Check sheet for the modelled part. Datum: model origin and axes. Units: mm. A direction names the side the tool comes from. Coordinates: 2 decimals unless noted, no trailing zeros. Write each loop counter-clockwise with the first axis right and the second up, starting at its lowest first coordinate (ties: lowest second). Pieces come first, ordered by that corner, then holes. Notation, with made-up numbers: (-2, -25) -> (11, -25) arc R19 cw to (11, 10) -> close; hole circle Ø3 at (80, 10.5). An arc over 180 degrees is marked (long way). Put each result on its own line as item: value.
```python
from build123d import *

# Parameters (mm, degrees)
SKETCH_1_R        = 19
SKETCH_1_R_2      = 17
EXTRUDE_2_DEPTH   = 11
EXTRUDE_2_2_DEPTH = 11
EXTRUDE_2_3_DEPTH = 11
EXTRUDE_2_4_DEPTH = 11
EXTRUDE_2_5_DEPTH = 11
EXTRUDE_2_6_DEPTH = 11
EXTRUDE_2_7_DEPTH = 11
EXTRUDE_2_8_DEPTH = 11
SKETCH_1_8_R      = 86
SKETCH_1_8_R_2    = 19
SKETCH_1_8_R_3    = 1.55
EXTRUDE_3_DEPTH   = 3


with BuildPart() as part:
    # Sketch 1 → Extrude 2 (new body)
    with BuildSketch(Plane(origin=(0, 0, 0), x_dir=(1, 0, 0), z_dir=(0, 1, 0))):
        with Locations(Location((-63, 0, 0), (0, 0, 270))):
            Circle(SKETCH_1_R)
        with Locations(Location((-63, 0, 0), (0, 0, 270))):
            Circle(SKETCH_1_R_2, mode=Mode.SUBTRACT)
    extrude(amount=EXTRUDE_2_DEPTH)



with BuildPart() as body_2:
    # Sketch 1 → Extrude 2 2 (new body)
    with BuildSketch(Plane(origin=(0, 0, 0), x_dir=(1, 0, 0), z_dir=(0, 1, 0))):
        with Locations(Location((-44.547727215, -44.547727215, 0), (0, 0, 270))):
            Circle(SKETCH_1_R)
        with Locations(Location((-44.547727215, -44.547727215, 0), (0, 0, 270))):
            Circle(SKETCH_1_R_2, mode=Mode.SUBTRACT)
    extrude(amount=EXTRUDE_2_2_DEPTH)


with BuildPart() as body_3:
    # Sketch 1 → Extrude 2 3 (new body)
    with BuildSketch(Plane(origin=(0, 0, 0), x_dir=(1, 0, 0), z_dir=(0, 1, 0))):
        with Locations(Location((0, -63, 0), (0, 0, 270))):
            Circle(SKETCH_1_R)
        with Locations(Location((0, -63, 0), (0, 0, 270))):
            Circle(SKETCH_1_R_2, mode=Mode.SUBTRACT)
    extrude(amount=EXTRUDE_2_3_DEPTH)


with BuildPart() as body_4:
    # Sketch 1 → Extrude 2 4 (new body)
    with BuildSketch(Plane(origin=(0, 0, 0), x_dir=(1, 0, 0), z_dir=(0, 1, 0))):
        with Locations(Location((44.547727215, -44.547727215, 0), (0, 0, 270))):
            Circle(SKETCH_1_R)
        with Locations(Location((44.547727215, -44.547727215, 0), (0, 0, 270))):
            Circle(SKETCH_1_R_2, mode=Mode.SUBTRACT)
    extrude(amount=EXTRUDE_2_4_DEPTH)


with BuildPart() as body_5:
    # Sketch 1 → Extrude 2 5 (new body)
    with BuildSketch(Plane(origin=(0, 0, 0), x_dir=(1, 0, 0), z_dir=(0, 1, 0))):
        with Locations(Location((63, 0, 0), (0, 0, 270))):
            Circle(SKETCH_1_R)
        with Locations(Location((63, 0, 0), (0, 0, 270))):
            Circle(SKETCH_1_R_2, mode=Mode.SUBTRACT)
    extrude(amount=EXTRUDE_2_5_DEPTH)


with BuildPart() as body_6:
    # Sketch 1 → Extrude 2 6 (new body)
    with BuildSketch(Plane(origin=(0, 0, 0), x_dir=(1, 0, 0), z_dir=(0, 1, 0))):
        with Locations(Location((0, 63, 0), (0, 0, 270))):
            Circle(SKETCH_1_R)
        with Locations(Location((0, 63, 0), (0, 0, 270))):
            Circle(SKETCH_1_R_2, mode=Mode.SUBTRACT)
    extrude(amount=EXTRUDE_2_6_DEPTH)


with BuildPart() as body_7:
    # Sketch 1 → Extrude 2 7 (new body)
    with BuildSketch(Plane(origin=(0, 0, 0), x_dir=(1, 0, 0), z_dir=(0, 1, 0))):
        with Locations(Location((44.547727215, 44.547727215, 0), (0, 0, 270))):
            Circle(SKETCH_1_R)
        with Locations(Location((44.547727215, 44.547727215, 0), (0, 0, 270))):
            Circle(SKETCH_1_R_2, mode=Mode.SUBTRACT)
    extrude(amount=EXTRUDE_2_7_DEPTH)


with BuildPart() as body_8:
    # Sketch 1 → Extrude 2 8 (new body)
    with BuildSketch(Plane(origin=(0, 0, 0), x_dir=(1, 0, 0), z_dir=(0, 1, 0))):
        with Locations(Location((-44.544339366, 44.544339366, 0), (0, 0, 270))):
            Circle(SKETCH_1_R)
        with Locations(Location((-44.544339366, 44.544339366, 0), (0, 0, 270))):
            Circle(SKETCH_1_R_2, mode=Mode.SUBTRACT)
    extrude(amount=EXTRUDE_2_8_DEPTH)


with BuildPart() as part_1:
    add(part.part)

    add(body_2.part)  # Extrude 3 merges body 2

    add(body_3.part)  # Extrude 3 merges body 3

    add(body_4.part)  # Extrude 3 merges body 4

    add(body_5.part)  # Extrude 3 merges body 5

    add(body_6.part)  # Extrude 3 merges body 6

    add(body_7.part)  # Extrude 3 merges body 7

    add(body_8.part)  # Extrude 3 merges body 8
    # Sketch 1_8 → Extrude 3 (add)
    with BuildSketch(Plane(origin=(0, 0, 0), x_dir=(1, 0, 0), z_dir=(0, 1, 0))):
        with Locations(Location((0, 0, 0), (0, 0, 270))):
            Circle(SKETCH_1_8_R)
        with Locations(Location((-63, 0, 0), (0, 0, 270))):
            Circle(SKETCH_1_8_R_2, mode=Mode.SUBTRACT)
        with Locations(Location((-44.547727215, -44.547727215, 0), (0, 0, 270))):
            Circle(SKETCH_1_8_R_2, mode=Mode.SUBTRACT)
        with Locations(Location((0, -63, 0), (0, 0, 270))):
            Circle(SKETCH_1_8_R_2, mode=Mode.SUBTRACT)
        with Locations(Location((44.547727215, -44.547727215, 0), (0, 0, 270))):
            Circle(SKETCH_1_8_R_2, mode=Mode.SUBTRACT)
        with Locations(Location((63, 0, 0), (0, 0, 270))):
            Circle(SKETCH_1_8_R_2, mode=Mode.SUBTRACT)
        with Locations(Location((44.547727215, 44.547727215, 0), (0, 0, 270))):
            Circle(SKETCH_1_8_R_2, mode=Mode.SUBTRACT)
        with Locations(Location((0, 63, 0), (0, 0, 270))):
            Circle(SKETCH_1_8_R_2, mode=Mode.SUBTRACT)
        with Locations(Location((-44.544339366, 44.544339366, 0), (0, 0, 270))):
            Circle(SKETCH_1_8_R_2, mode=Mode.SUBTRACT)
        with Locations(Location((0, -7, 0), (0, 0, 270))):
            Circle(SKETCH_1_8_R_3, mode=Mode.SUBTRACT)
        with Locations(Location((-7, 0, 0), (0, 0, 270))):
            Circle(SKETCH_1_8_R_3, mode=Mode.SUBTRACT)
        with Locations(Location((7, 0, 0), (0, 0, 270))):
            Circle(SKETCH_1_8_R_3, mode=Mode.SUBTRACT)
        with Locations(Location((0, 7, 0), (0, 0, 270))):
            Circle(SKETCH_1_8_R_3, mode=Mode.SUBTRACT)
        with Locations(Location((0, 0, 0), (0, 0, 270))):
            Circle(SKETCH_1_8_R_3, mode=Mode.SUBTRACT)
    extrude(amount=EXTRUDE_3_DEPTH)


solid = part_1.part
```
Q1. Cross-section at C-C (x = 30). Record the cut outline in (y, z), plus the area to 3 significant figures.
Recorded:
outline: (0, -80.6) -> (3, -80.6) -> (3, -56.77) -> (11, -56.77) -> (11, -53.34) -> (0, -53.34) -> close; (0, -35.75) -> (11, -35.75) -> (11, -32.33) -> (3, -32.33) -> (3, 32.33) -> (11, 32.33) -> (11, 35.75) -> (0, 35.75) -> close; (0, 53.34) -> (11, 53.34) -> (11, 56.77) -> (3, 56.77) -> (3, 80.6) -> (0, 80.6) -> close
area: 488 mm2
Q2. Material ranges on line 1 along X through (y, z) = (1.75, 35); line 2 along X through (y, z) = (9, 7.5); line 3 along X through (y, z) = (5.5, -29), recorded low to high.
Recorded:
line 1: x = -78.56 to -58.61, -30.48 to 30.48, 58.61 to 78.56
line 2: x = -80.46 to -78.26, -47.74 to -45.54, 45.54 to 47.74, 78.26 to 80.46
line 3: x = -55.47 to -51.43, -37.66 to -33.62, 33.63 to 37.67, 51.42 to 55.47
Q3. Cross-section at D-D (x = -57). Record the cut outline in (y, z), plus the area to 3 significant figures.
Recorded:
outline: (0, -64.4) -> (3, -64.4) -> (3, -58.89) -> (11, -58.89) -> (11, -56.11) -> (0, -56.11) -> close; (0, -32.97) -> (11, -32.97) -> (11, -30.2) -> (3, -30.2) -> (3, -18.03) -> (11, -18.03) -> (11, -15.91) -> (0, -15.91) -> close; (0, 15.91) -> (11, 15.91) -> (11, 18.03) -> (3, 18.03) -> (3, 30.2) -> (11, 30.2) -> (11, 32.97) -> (0, 32.97) -> close; (0, 56.12) -> (11, 56.12) -> (11, 58.9) -> (3, 58.9) -> (3, 64.4) -> (0, 64.4) -> close
area: 275 mm2
Q4. Depth check by flat-ended pin: P1, Ø3.5, axis at x = 0, z = 7, coming from the +Y side; P2, Ø3.5, axis at x = -7, z = 0, coming from the -Y side; P3, Ø6, axis at y = 1.5, z = -45, coming from the +X side; P4, Ø1.5, axis at y = 9, z = 35.5, coming from the +X side. Enter the tip coordinate at first touch or a pass-through.
Recorded:
P1: stops at y = 3
P2: stops at y = 0
P3: stops at x = 75.05
P4: stops at x = 61.64
Q5. Mould release check, pull along X, two halves, no side actions. Record for faces 3 (the cylindrical face through (57.389, 6.944, 30.544)), 4 (the cylindrical face through (57.39, 6.94, -58.55)), 5 (the flat face through (35, 11, 30)): released by +X, released by -X, zero draft, split by the parting line, or undercut.
Recorded:
face 3: undercut
face 4: undercut
face 5: zero draft
Q6. Cross-section at B-B (z = -70.5). Record the cut outline in (x, y).
Recorded:
outline: (-49.25, 0) -> (-15.26, 0) -> (-15.26, 11) -> (-17.46, 11) -> (-17.46, 3) -> (-49.25, 3) -> close; (15.26, 0) -> (49.25, 0) -> (49.25, 3) -> (17.46, 3) -> (17.46, 11) -> (15.26, 11) -> close
Q7. Tool access check on faces 1 (the cylindrical face through (-43.8, 5.423, 27.564)), 2 (the cylindrical face through (79.021, 6.944, 10.214)). Record the directions out of +Z, -Z, +X, -X, +Y, -Y that give a thin tool (end or side, any length) a straight path to the whole face; none if there is none.
Recorded:
face 1: +Y, -Y
face 2: +Y
Q8. Cross-section at A-A (y = 6.5). State how many separate pieces and enclosed holes the cut face has, plus the area to 3 significant figures.
Recorded:
separate pieces: 8
enclosed holes: 8
area: 1,810 mm2
